Work out the finished part from the listing and answer in its coordinate system (mm). A direction names the side the tool comes from. Give positions to 0.01 mm unless a question says otherwise; leave off trailing zeros. Write each loop counter-clockwise with the first axis right and the second up, starting at its lowest first coordinate (ties: lowest second). Pieces come first, ordered by that corner, then holes. Notation, with made-up numbers: (-2, 39.5) -> (27, 39.5) arc R36 ccw to (27, 74.5) -> close; hole circle Ø7 at (81.5, -8.75). An arc over 180 degrees is marked (long way). Write item = value, one per line. Start each with the question number.
Autodesk Inventor part; units mm, degrees
ref_plane "YZ Plane" through (0, 0, 0) normal (1, 0, 0) x (0, 1, 0)
ref_plane "XZ Plane" through (0, 0, 0) normal (0, 1, 0) x (-1, 0, 0)
ref_plane "XY Plane" through (0, 0, 0) normal (0, 0, 1) x (1, 0, 0)
sketch "Sketch1" plane through (0, 0, 0) normal (0, 1, 0) x (-1, 0, 0)
  line L0 (45, -40) -> (-45, -40)
  line L1 (-45, -40) -> (-45, 40)
  line L2 (-45, 40) -> (45, 40)
  line L3 (45, 40) -> (45, -40)
  line L4 (45, -40) -> (-45, 40) construction
  line L5 (-45, -40) -> (45, 40) construction
  point P0 (0, 0)
  dimension "d0" = 90
  dimension "d1" = 80
extrude "Extrusion1" add sketch "Sketch1" along normal blind 38
sketch "Sketch2" plane through (0, 38, 0) normal (0, 1, 0) x (1, 0, 0)
  line L0 (-45, -40) -> (45, -40)
  line L1 (45, -40) -> (45, 40)
  line L2 (45, 40) -> (-45, 40)
  line L3 (-45, 40) -> (-45, -40)
  line L4 (-25.1, 40) -> (25.1, 40)
  line L5 (25.1, 40) -> (25.1, 20)
  line L6 (25.1, 20) -> (-25.1, 20)
  line L7 (-25.1, 20) -> (-25.1, 40)
  line L8 (-25.1, 20) -> (25.1, 20)
  line L9 (25.1, 20) -> (25.1, -30)
  line L10 (25.1, -30) -> (-25.1, -30)
  line L11 (-25.1, -30) -> (-25.1, 20)
  point P0 (0, 0)
  point P1 (0, 40)
  dimension "d4" = 50.2
  dimension "d5" = 20
  dimension "d24" = 50
extrude "Extrusion2" cut sketch "Sketch2" against normal blind 27.5 contours L2 L5 L6 L7 | L6 L9 L10 L11
sketch "Sketch3" plane through (-45, 0, 40) normal (0, 0, 1) x (1, 0, 0)
  circle A0 centre (32.5, 33) radius 2.067 construction
  circle A1 centre (57.5, 33) radius 2.067 construction
  line L0 (0, 0) -> (90, 0) construction
  line L1 (90, 0) -> (90, 38) construction
  line L2 (0, 38) -> (90, 38) construction
  line L3 (0, 0) -> (0, 38) construction
  line L4 (0, 15) -> (90, 15) construction
  line L5 (45, 0) -> (45, 38) construction
  point P0 (10, 15)
  point P1 (80, 15)
  dimension "d8" = 15
  dimension "d9" = 10
hole "Hole1" at (-12.5, 33, 40) at (12.5, 33, 40) direction (0, 0, -1) diameter 5.2 end through all
sketch "Sketch4" plane through (-45, 0, 40) normal (0, 0, 1) x (1, 0, 0)
  point P0 (45, 0)
  point P1 (10.0426, 14.4118)
  point P2 (80.769, 14.5558)
hole "Hole2" at (-34.9574, 14.4118, 40) at (35.769, 14.5558, 40) direction (0, 0, -1) diameter 5.2 end through all counterbore diameter 10 counterbore depth 48
fillet "Fillet1" radius 3 4 edges at (-45, 19, 40) (45, 19, 40) (35.05, 38, -40) (-35.05, 38, -40)
properties part number "T-Frame_encoder_frame" material "ABS Plastic"
(1) Determine the mould class of faces 1 (the cylindrical face through (-44.14, 19.27, 39.1)), 2 (the cylindrical face through (14.082, 35.063, 34.93)), 3 (the flat face through (1, 0, 1)), 4 (the cylindrical face through (-37.535, 14.75, -24.224)) for opening direction X: pulls with the +X half, pulls with the -X half, needs draft (parallel to the pull), parting line crosses it, or undercut.
(2) A cutting plane is placed at D-D, the plane y = 27. Write down the section's boundary in (x, z).
(3) A cutting plane is placed at B-B, the plane x = 12.5. Write down the section's boundary in (y, z).
(4) A cutting plane is placed at C-C, the plane z = 0.5. Write down the section's boundary in (x, y).
(5) For faces 5 (the cylindrical face through (44.1, 19.27, 39.14)), 6 (the cylindrical face through (-36.459, 9.643, 15.664)), 7 (the flat face through (0, 24, 30)), determine the directions among +Z, -Z, +X, -X, +Y, -Y from which every point of the face is accessible in a straight line to the end or side of a thin tool.
(6) A cutting plane is placed at A-A, the plane y = 33. Write down the section's boundary in (x, z), then the cut area to 3 significant figures.
(7) Find the intervals of material crossed by line 1 along X through (y, z) = (33, 32.25); line 2 along X through (y, z) = (20, 25.5); line 3 along X through (y, z) = (16, 25.5), in increasing order.
(8) Each of these flat-tipped pins is pushed along its axis until it touches: pin 1 (3 mm diameter, centred on x = -5, z = 17, fed in from +Y); pin 2 (11 mm diameter, centred on x = -34.5, y = 16, fed in from +Z); pin 3 (8.5 mm diameter, centred on x = 12.5, y = 33, fed in from -Z); pin 4 (8.5 mm diameter, centred on x = 35.77, y = 14.56, fed in from +Z). Where does it stop, or does it pass through?
Results list:
q1.face_1 = pulls with the -X half
q1.face_2 = undercut
q1.face_3 = needs draft
q1.face_4 = undercut
q2.outline = (-45, -40) -> (-25.1, -40) -> (-25.1, 30) -> (25.1, 30) -> (25.1, -40) -> (45, -40) -> (45, 37) arc R3 ccw to (42, 40) -> (-42, 40) arc R3 ccw to (-45, 37) -> close
q3.outline = (0, -40) -> (10.5, -40) -> (10.5, 30) -> (30.4, 30) -> (30.4, 40) -> (0, 40) -> close; (35.6, 30) -> (38, 30) -> (38, 40) -> (35.6, 40) -> close
q4.outline = (-45, 0) -> (45, 0) -> (45, 38) -> (25.1, 38) -> (25.1, 10.5) -> (-25.1, 10.5) -> (-25.1, 38) -> (-45, 38) -> close; hole circle Ø10 at (-34.96, 14.41); hole circle Ø10 at (35.77, 14.56)
q5.face_5 = +Z, +X, +Y, -Y
q5.face_6 = +Z
q5.face_7 = -Z, +Y
q6.outline = (-45, -40) -> (-25.1, -40) -> (-25.1, 30) -> (-15.1, 30) -> (-15.1, 40) -> (-42, 40) arc R3 ccw to (-45, 37) -> close; (-9.9, 30) -> (9.9, 30) -> (9.9, 40) -> (-9.9, 40) -> close; (15.1, 30) -> (25.1, 30) -> (25.1, -40) -> (45, -40) -> (45, 37) arc R3 ccw to (42, 40) -> (15.1, 40) -> close
q6.area = 3,580 mm²
q7.line_1 = -45 to -15.1, -9.9 to 9.9, 15.1 to 45
q7.line_2 = -45 to -25.1, 25.1 to 45
q7.line_3 = -45 to -39.7, -30.22 to -25.1, 25.1 to 30.98, 40.56 to 45
q8.pin_1 = 10.5
q8.pin_2 = 40
q8.pin_3 = 30
q8.pin_4 = -8
